Geometry check sheet. Reference: the model listing, model coordinates, mm. A direction names the side the tool comes from. Round coordinates to 2 decimals unless told otherwise and drop trailing zeros. Order: outer loops, then holes, each group sorted by start corner. A loop starts at its lowest first (then second) coordinate and runs counter-clockwise, first axis right, second up.
(1) Thickness scan on L1, parallel to X at y = 8.5, z = 28.5; L2, parallel to Z at x = 20, y = -0.5 (3 decimals); L3, parallel to Y at x = -5.5, z = 10. Record the ranges inside material, lowest first.
(2) Cross-section at D-D on x = 2.5. Enter the section's corners in (y, z).
(3) Draft check along Z on faces 1 (the face through (10.85, -5.81, 1.73)), 2 (the face through (0, 2, 0)), 3 (the face through (11, -8, 30)), 4 (the face through (11, 2, -20)). Enter one of: pulls with the +Z half, pulls with the -Z half, needs draft (parallel to the pull), parting line crosses it, or undercut.
(4) Cross-section at A-A on x = -8. Enter the section's corners in (y, z), and give its area (3 significant figures).
(5) Set-up check for faces 5 (the face through (6, -18, -20)), 6 (the face through (11, -8, -31)), 7 (the face through (0, 18, -8)): record each of +Z, -Z, +X, -X, +Y, -Y from which the full face is reachable in a straight line by a thin tool's end or side.
(6) Cross-section at C-C on z = 0. Enter the section's corners in (x, y).
(7) Gauge pin test, flat ends, axial feed: P1, Ø10, axis at x = 13.5, z = -10.5, coming from the +Y side (3 decimals); P2, Ø2, axis at x = 10, z = 14, coming from the -Y side; P3, Ø0.9, axis at x = 5.5, z = -30.5, coming from the +Y side. Record the tip position at first contact, or that the pin passes through.
(8) Cross-section at B-B on y = 2. Enter the section's corners in (x, z), and give its area (3 significant figures).
from build123d import *

# Parameters (mm, degrees)
SKETCH1_R           = 8
BOSS_EXTRUDE2_DEPTH = 22
SKETCH2_R           = 8
SKETCH2_W           = 16
SKETCH2_H           = 9
BOSS_EXTRUDE4_DEPTH = 10


with BuildPart() as part:
    # Sketch1 → Boss-Extrude2 (new body)
    with BuildSketch(Plane(origin=(0, 0, 0), x_dir=(0, 0, -1), z_dir=(1, 0, 0))):
        with BuildLine():
            Line((32, -8), (29, -8))
            ThreePointArc((29, -8), (27.658359214, -7.683281573), (26.6, -6.8))
            Line((26.6, -6.8), (12.8, 11.6))
            ThreePointArc((12.8, 11.6), (0, 18), (-12.8, 11.6))
            Line((-12.8, 11.6), (-26.6, -6.8))
            ThreePointArc((-26.6, -6.8), (-27.658359214, -7.683281573), (-29, -8))
            Line((-29, -8), (-32, -8))
            Line((-32, -8), (-32, -18))
            Line((-32, -18), (-8, -18))
            Line((-8, -18), (-8, -27))
            Line((-8, -27), (8, -27))
            Line((8, -27), (8, -18))
            Line((8, -18), (32, -18))
            Line((32, -18), (32, -8))
        make_face()
        with Locations((0, 2)):
            Circle(SKETCH1_R, mode=Mode.SUBTRACT)
    extrude(amount=BOSS_EXTRUDE2_DEPTH)

    # Sketch2 → Boss-Extrude4 (add)
    with BuildSketch(Plane.ZY):
        with BuildLine():
            Line((-32, 23.051846753), (-32, -8))
            Line((-32, -8), (-29, -8))
            ThreePointArc((-29, -8), (-27.658359214, -7.683281573), (-26.6, -6.8))
            Line((-26.6, -6.8), (-12.8, 11.6))
            ThreePointArc((-12.8, 11.6), (0, 18), (12.8, 11.6))
            Line((12.8, 11.6), (26.6, -6.8))
            ThreePointArc((26.6, -6.8), (27.658359214, -7.683281573), (29, -8))
            Line((29, -8), (32, -8))
            Line((32, -8), (32, 23.051846753))
            Line((32, 23.051846753), (-32, 23.051846753))
        make_face()
        with BuildLine():
            Line((-32, -18), (-8, -18))
            Line((-8, -18), (8, -18))
            Line((8, -18), (32, -18))
            Line((32, -18), (32, -8))
            Line((32, -8), (29, -8))
            ThreePointArc((29, -8), (27.658359214, -7.683281573), (26.6, -6.8))
            Line((26.6, -6.8), (12.8, 11.6))
            ThreePointArc((12.8, 11.6), (0, 18), (-12.8, 11.6))
            Line((-12.8, 11.6), (-26.6, -6.8))
            ThreePointArc((-26.6, -6.8), (-27.658359214, -7.683281573), (-29, -8))
            Line((-29, -8), (-32, -8))
            Line((-32, -8), (-32, -18))
        make_face()
        with Locations((0, 2)):
            Circle(SKETCH2_R, mode=Mode.SUBTRACT)
        with Locations((0, -22.5)):
            Rectangle(SKETCH2_W, SKETCH2_H)
        with Locations((0, 2)):
            Circle(SKETCH2_R)
    extrude(amount=BOSS_EXTRUDE4_DEPTH)


solid = part.part
Found:
1. L1: x = -10 to 0
1. L2: z = -21.875 to -7.599, 7.599 to 21.875
1. L3: y = -18 to 23.05
2. outline: (-27, -8) - (-18, -8) - (-18, -32) - (-8, -32) - (-8, -29) arc R3 cw to (-6.8, -26.6) - (11.6, -12.8) arc R16 ccw to (11.6, 12.8) - (-6.8, 26.6) arc R3 cw to (-8, 29) - (-8, 32) - (-18, 32) - (-18, 8) - (-27, 8) - close; hole circle Ø16 at (2, 0)
3. face 1: undercut
3. face 2: undercut
3. face 3: needs draft
3. face 4: pulls with the -Z half
4. outline: (-27, -8) - (-18, -8) - (-18, -32) - (23.05, -32) - (23.05, 32) - (-18, 32) - (-18, 8) - (-27, 8) - close
4. area: 2,770 mm2
5. face 5: -Z, +X, -X, -Y
5. face 6: -Z, +X, +Y
5. face 7: +X, +Y
6. outline: (-10, -27) - (22, -27) - (22, -6) - (0, -6) - (0, 10) - (22, 10) - (22, 18) - (0, 18) - (0, 23.05) - (-10, 23.05) - close
7. P1: stops at y = 17.025
7. P2: stops at y = -18
7. P3: stops at y = -8
8. outline: (-10, -32) - (0, -32) - (0, -20) - (22, -20) - (22, -8) - (0, -8) - (0, 8) - (22, 8) - (22, 20) - (0, 20) - (0, 32) - (-10, 32) - close
8. area: 1,170 mm2
